from build123d import *

# Parameters (mm, degrees)
SKETCH1_W           = 15.9004
SKETCH1_H           = 11.938
BOSS_EXTRUDE1_DEPTH = 17.526
SHELL1_T            = -1.27
SKETCH2_W           = 1.905
SKETCH2_H           = 3.5052
BOSS_EXTRUDE2_DEPTH = 0.254


with BuildPart() as part:
    # Sketch1 → Boss-Extrude1 (new body)
    with BuildSketch(Plane.XY):
        Rectangle(SKETCH1_W, SKETCH1_H)
    extrude(amount=-BOSS_EXTRUDE1_DEPTH)

    # Shell1
    shell1_openings = [part.faces().sort_by_distance(p)[0] for p in [
        (0, 0, 0),
    ]]
    offset(amount=SHELL1_T, openings=shell1_openings, kind=Kind.INTERSECTION)

    # Sketch2 → Boss-Extrude2 (add)
    with BuildSketch(Plane.XZ.offset(5.969)):
        with Locations((-8.9027, -5.461)):
            Rectangle(SKETCH2_W, SKETCH2_H)
    boss_extrude2 = extrude(amount=-BOSS_EXTRUDE2_DEPTH)

    # Mirror1: Boss-Extrude2 across plane
    add(boss_extrude2.mirror(Plane(origin=(0, 0, 0), x_dir=(0, 0, 1), z_dir=(1, 0, 0))))


solid = part.part
Could you check a few things on this model? Use its own coordinates, in mm. A direction names the side the tool comes from. Give positions to 0.01 mm unless a question says otherwise; leave off trailing zeros. Order: outer loops, then holes, each group sorted by start corner. A loop starts at its lowest first (then second) coordinate and runs counter-clockwise, first axis right, second up. Notation, with made-up numbers: M 23.25,49.5 L 29.25,49.5 A5 cw 29.25,54.5 Z; hole C 65,59 d5. An arc over 180 degrees is marked long. One line per question, with ' | ' between items.
1. I want a section at D-D (z = -4). List the corners of the cut face in (x, y) for me (3 decimals).
Results:
outline: M -9.855,-5.969 L 9.855,-5.969 L 9.855,-5.715 L 7.95,-5.715 L 7.95,5.969 L -7.95,5.969 L -7.95,-5.715 L -9.855,-5.715 Z; hole M -6.68,-4.699 L 6.68,-4.699 L 6.68,4.699 L -6.68,4.699 Z
2. I want a section at B-B (x = 0.25). List the corners of the cut face in (y, z) for me.
Results:
outline: M -5.97,-17.53 L 5.97,-17.53 L 5.97,0 L 4.7,0 L 4.7,-16.26 L -4.7,-16.26 L -4.7,0 L -5.97,0 Z
3. For faces 4 (the face through (0, -4.699, -8)), 5 (the face through (-9, -5.715, -5)), 6 (the face through (9, -5.715, -5)), which set-ups out of +Z, -Z, +X, -X, +Y, -Y let a thin tool reach every point of the face, with its end or its side?
Results:
face 4: +Z | face 5: +Z, -Z, -X, +Y | face 6: +Z, -Z, +X, +Y
4. If I drill on line 1 (Y direction, x = 0.5, z = -14); line 2 (X direction, y = -0.5, z = -13.25); line 3 (Z direction, x = 2, y = 0.75), over which ranges is the centre line in solid material (lowest first)?
Results:
line 1: -5.97 to -4.7, 4.7 to 5.97 | line 2: -7.95 to -6.68, 6.68 to 7.95 | line 3: -17.53 to -16.26
5. We'd pull the mould along Y, two halves only. Please class faces 1 (the face through (0, -5.969, -9)), 2 (the face through (0, 5.969, -9)), 3 (the face through (6.68, 0, -8)): +Y half, -Y half, draft (parallel to the pull), parting line (faces both ways), or undercut.
Results:
face 1: -Y half | face 2: +Y half | face 3: undercut
6. I'm going to push flat-ended pins straight in: pin 1 (1 mm diameter, centred on y = 4, z = -8.5, fed in from -X); pin 2 (4 mm diameter, centred on y = -0.5, z = -13.5, fed in from +X); pin 3 (1 mm diameter, centred on x = 8.5, z = -5.5, fed in from +Y) (3 decimals). Where does each tip first touch, or does it pass through?
Results:
pin 1: x = -7.95 | pin 2: x = 7.95 | pin 3: y = -5.715
7. I want a section at C-C (y = -1.5). List the corners of the cut face in (x, z) for me.
Results:
outline: M -7.95,-17.53 L 7.95,-17.53 L 7.95,0 L 6.68,0 L 6.68,-16.26 L -6.68,-16.26 L -6.68,0 L -7.95,0 Z
8. I want a section at A-A (z = -8.5). List the corners of the cut face in (x, y) for me.
Results:
outline: M -7.95,-5.97 L 7.95,-5.97 L 7.95,5.97 L -7.95,5.97 Z; hole M -6.68,-4.7 L 6.68,-4.7 L 6.68,4.7 L -6.68,4.7 Z
